from build123d import *

# Parameters (mm, degrees)
F0_W     = 15.24
F0_H     = 15.24
F0_R     = 3.4925
F0_R_2   = 2.2225
F1_DEPTH = 1.27
F0_W_2   = 17.78
F0_H_2   = 17.78
F2_DEPTH = 12.7
F3_DEPTH = 12.7


with BuildPart() as f1:
    # F0 (on Top) → F1 (new body)
    with BuildSketch(Plane.XY):
        Rectangle(F0_W, F0_H)
        Circle(F0_R, mode=Mode.SUBTRACT)
        Circle(F0_R)
        Circle(F0_R_2, mode=Mode.SUBTRACT)
        Circle(F0_R_2)
    extrude(amount=F1_DEPTH)

    # F0 (on Top) → F2 (join)
    with BuildSketch(Plane.XY):
        Rectangle(F0_W_2, F0_H_2)
        Rectangle(F0_W, F0_H, mode=Mode.SUBTRACT)
    extrude(amount=F2_DEPTH)

    # F0 (on Top) → F3 (join)
    with BuildSketch(Plane.XY):
        Circle(F0_R)
        Circle(F0_R_2, mode=Mode.SUBTRACT)
    extrude(amount=F3_DEPTH)


solid = f1.part
Input: part model. Units: mm. Frame: model coordinates. A direction names the side the tool comes from. Give positions to 0.01 mm unless a question says otherwise; leave off trailing zeros. Order: outer loops, then holes, each group sorted by start corner. A loop starts at its lowest first (then second) coordinate and runs counter-clockwise, first axis right, second up.
Q1. Section C-C on y = -4.25. Output: boundary loops of the cut face in (x, z).
Checked values:
outline: (-8.89, 0) - (8.89, 0) - (8.89, 12.7) - (7.62, 12.7) - (7.62, 1.27) - (-7.62, 1.27) - (-7.62, 12.7) - (-8.89, 12.7) - close
Q2. Ray query, probe 1 along X at (y, z) = (0, 7.25); probe 2 along Y at (x, z) = (0.75, 1.75). Return the intervals inside material, ascending.
Checked values:
probe 1: x = -8.89 to -7.62, -3.49 to -2.22, 2.22 to 3.49, 7.62 to 8.89
probe 2: y = -8.89 to -7.62, -3.41 to -2.09, 2.09 to 3.41, 7.62 to 8.89
Q3. Contact query for flat-ended pins moving along their axis: pin 1 Ø5 at (x, y) = (0.5, -0.5) entering from +Z; pin 2 Ø4 at (x, y) = (0, 0) entering from +Z. Output: stop coordinate, or through.
Checked values:
pin 1: stops at z = 12.7
pin 2: stops at z = 1.27
Q4. Section B-B on x = 0. Output: boundary loops of the cut face in (y, z), and give its area (3 significant figures).
Checked values:
outline: (-8.89, 0) - (8.89, 0) - (8.89, 12.7) - (7.62, 12.7) - (7.62, 1.27) - (3.49, 1.27) - (3.49, 12.7) - (2.22, 12.7) - (2.22, 1.27) - (-2.22, 1.27) - (-2.22, 12.7) - (-3.49, 12.7) - (-3.49, 1.27) - (-7.62, 1.27) - (-7.62, 12.7) - (-8.89, 12.7) - close
area: 80.6 mm2
Q5. Set-up query: faces 4 (the flat face through (0, 0, 1.27)), 5 (the flat face through (-8.89, 0, 6)). Return all of +Z, -Z, +X, -X, +Y, -Y with unobstructed straight access to the full face (end or side cutting, diameter ignored); none if empty.
Checked values:
face 4: +Z
face 5: +Z, -Z, -X, +Y, -Y
Q6. Draft query along Y for faces 1 (the flat face through (0, 8.89, 6)), 2 (the flat face through (0.7, -2.3, 12.7)), 3 (the flat face through (-1.8, 3.5, 1.27)). Return one class per face: +Y half, -Y half, draft (parallel to the pull), parting line (faces both ways), or undercut.
Checked values:
face 1: +Y half
face 2: draft
face 3: undercut
Q7. Section A-A on z = 10. Output: boundary loops of the cut face in (x, y) (1 decimal), and give its area (3 significant figures).
Checked values:
outline: (-8.9, -8.9) - (8.9, -8.9) - (8.9, 8.9) - (-8.9, 8.9) - close; circle Ø7 at (0, 0); hole (-7.6, -7.6) - (7.6, -7.6) - (7.6, 7.6) - (-7.6, 7.6) - close; hole circle Ø4.4 at (0, 0)
area: 107 mm2
